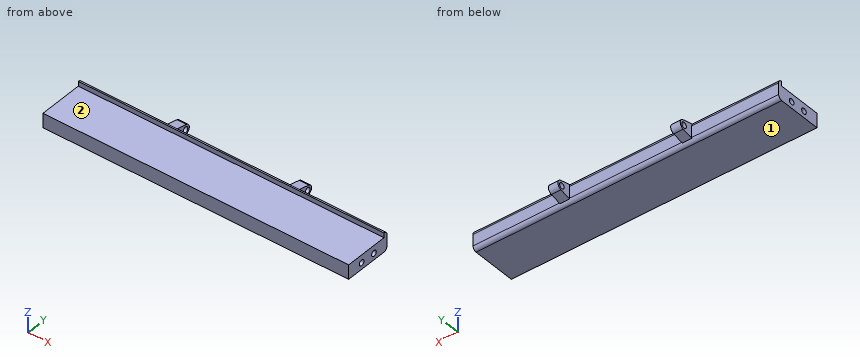
Autodesk Inventor part; units mm, degrees
ref_plane "Work Plane1" through (-8, -12.5, 0) normal (1, 0, 0) x (0, 0, -1)
ref_plane "Work Plane2" through (-40, -12.5, 0) normal (-1, 0, 0) x (0, 0, 1)
ref_plane "Work Plane3" through (20, 10.5, 6) normal (0, 0, -1) x (-1, 0, 0)
sketch "Sketch1" plane through (0, 0, 0) normal (0, 0, 1) x (1, 0, 0)
  line L0 (40, 12.5) -> (-40, 12.5)
  line L1 (-40, 12.5) -> (-40, -12.5)
  line L2 (-40, -12.5) -> (40, -12.5)
  line L3 (40, -12.5) -> (40, 12.5)
  line L4 (40, 12.5) -> (-40, -12.5) construction
  line L5 (-40, 12.5) -> (40, -12.5) construction
  point P0 (0, 0)
  dimension "d0" = 80
  dimension "d1" = 25
extrude "Extrusion1" add sketch "Sketch1" along normal blind 10
ref_plane "Work Plane1" through (-8, -12.5, 0) normal (1, 0, 0) x (0, 0, -1)
sketch "Sketch2" plane through (-8, -12.5, 0) normal (1, 0, 0) x (0, 0, -1)
  circle A0 centre (-5.3658, 30) radius 2.5
  line L0 (0, 25) -> (-10, 25)
  line L1 (-9.1092, 25) -> (-7.7995, 30.572)
  line L2 (-2.9321, 30.572) -> (-1.6224, 25)
  point P0 (0, 12.5)
  dimension "d5" = 5
  dimension "d11" = 5
extrude "Extrusion2" add sketch "Sketch2" along normal mid plane 5
sketch "Sketch3" plane through (-5.5, -12.5, 0) normal (1, 0, 0) x (0, 0, -1)
  arc A0 (-2.9321, 30.572) -> (-7.7995, 30.572) centre (-5.3658, 30) ccw
  circle A1 centre (-5.3658, 30) radius 1.5
  point P0 (0, 12.5)
  dimension "d8" = 3
extrude "Extrusion3" cut sketch "Sketch3" against normal blind 20
sketch "Sketch4" plane through (0, 0, 0) normal (0, 0, -1) x (-1, 0, 0)
  point P0 (0, 0)
sketch "Sketch5" plane through (-40, -12.5, 0) normal (-1, 0, 0) x (0, 0, 1)
  point P0 (0, 12.5)
ref_plane "Work Plane2" through (-40, -12.5, 0) normal (-1, 0, 0) x (0, 0, 1)
mirror "Mirror1" about plane through (-40, 12.5, 0) normal (-1, 0, 0) of "Extrusion2", "Extrusion1"
fillet "Fillet1" radius 2 2 edges at (-40, 12.5, 10) (-40, 12.5, 0)
sketch "Sketch6" plane through (-74.5, 17.5, 5.3658) normal (-1, 0, 0) x (0, 0, 1)
  circle A0 centre (0, 0) radius 1.5
  point P0 (-5.3658, -17.5)
extrude "Extrusion4" cut sketch "Sketch6" against normal blind 20
ref_plane "Work Plane3" through (20, 10.5, 6) normal (0, 0, -1) x (-1, 0, 0)
sketch "Sketch7" plane through (40, -12.5, 10) normal (1, 0, 0) x (0, 0, -1)
  circle A0 centre (6.606, 16.5) radius 1.5
  circle A1 centre (6.606, 8.5) radius 1.5
  line L0 (10, 0) -> (0, 0)
  line L1 (10, 0) -> (10, 23)
  point P0 (10, 12.5)
  point P1 (5, 0)
  dimension "d16" = 3
  dimension "d17" = 3
  dimension "d19" = 8.5
  dimension "d20" = 8
  dimension "d32" = 3.394
  dimension "d33" = 3.394
extrude "Extrusion5" cut sketch "Sketch7" against normal blind 8
ref_plane "Work Plane4" through (-120, -12.5, 0) normal (-1, 0, 0) x (0, 0, 1)
mirror "Mirror2" about plane through (-40, -12.5, 0) normal (-1, 0, 0) of "Extrusion5"
thread "Thread1"
thread "Thread2"
thread "Thread3"
thread "Thread4"
sketch "Sketch8" plane through (0, 0, 0) normal (0, 0, -1) x (-1, 0, 0)
  line L0 (-40, 10.5) -> (120, 10.5) construction
  line L1 (-40, -12.5) -> (-40, 10.5) construction
  line L2 (-40, -12.5) -> (120, -12.5) construction
  line L3 (120, -12.5) -> (120, 10.5)
  point P0 (0, 0)
sketch "Sketch9" plane through (0, 0, 10) normal (0, 0, 1) x (1, 0, 0)
  line L0 (-120, 10.5) -> (40, 10.5)
  line L1 (-120, -12.5) -> (-120, 10.5)
  line L2 (40, -12.5) -> (-120, -12.5)
  line L3 (40, -12.5) -> (40, 10.5)
  point P0 (0, 0)
extrude "Extrusion6" cut sketch "Sketch9" against normal blind 2.5
properties part number "plate"
Can you work these out from the model? Positions are in its coordinate system, mm. Face numbers are marked on the shaded views. A direction names the side the tool comes from. Coordinates: 2 decimals unless noted, no trailing zeros. Order: outer loops, then holes, each group sorted by start corner. A loop starts at its lowest first (then second) coordinate and runs counter-clockwise, first axis right, second up. Notation, with made-up numbers: (55.25, 84) - (103.25, 84) arc R20 ccw to (103.25, 94) - close; hole circle Ø10 at (-30.5, 49.25). An arc over 180 degrees is marked (long way). Answer as a JSON object with one key per item and string values. Group by question number.
Q1. Imagine slicing it at A-A (x = -30). Please give me the cut outline in (y, z).
Q2. Will these pins go through, and if not, where does the flat tip stop? P1, Ø6, axis at y = 16.5, z = 5, coming from the -X side; P2, Ø0.9, axis at y = -4, z = 3, coming from the -X side; P3, Ø1.8, axis at y = -4, z = 3.394, coming from the +X side.
Q3. On a 3-axis mill with a long thin cutter (end or side, diameter ignored), from which of +Z, -Z, +X, -X, +Y, -Y can I reach the whole of each face in a straight line? I mean the marked faces 1 and 2. Say none if no direction works.
Q4. I need wall thicknesses on line 1 (Z direction, x = -74.5, y = -9); line 2 (Z direction, x = -72, y = 17); line 3 (Y direction, x = -111, z = 6.5). Which ranges of each line are inside material? Lowest first, please. Write a range as from..to.
Q5. Imagine slicing it at B-B (y = -4). Please give me the cut outline in (x, z), and give its area (3 significant figures).
Q6. Imagine slicing it at C-C (x = -7). Please give me the cut outline in (y, z).
Determined:
{
 "1": {"outline": "(-12.5, 0) - (10.5, 0) arc R2 ccw to (12.5, 2) - (12.5, 8) arc R2 ccw to (10.5, 10) - (10.5, 7.5) - (-12.5, 7.5) - close"},
 "2": {"P1": "stops at x = -74.5", "P2": "stops at x = -112", "P3": "stops at x = 32"},
 "3": {"face 1": "-Z, +X, -X, +Y, -Y", "face 2": "+Z, +X, -X, -Y"},
 "4": {"line 1": "z = 0..7.5", "line 2": "z = 2.68..3.95, 6.78..8.05", "line 3": "y = -12.5..12.5"},
 "5": {"outline": "(-120, 0) - (40, 0) - (40, 1.89) - (32, 1.89) - (32, 4.89) - (40, 4.89) - (40, 7.5) - (-120, 7.5) - (-120, 4.89) - (-112, 4.89) - (-112, 1.89) - (-120, 1.89) - close", "area": "1,150 mm2"},
 "6": {"outline": "(-12.5, 0) - (10.5, 0) arc R2 ccw to (12.46, 1.61) - (18.07, 2.93) arc R2.5 ccw to (18.07, 7.8) - (12.1, 9.2) arc R2 ccw to (10.5, 10) - (10.5, 7.5) - (-12.5, 7.5) - close; hole circle Ø3 at (17.5, 5.37)"}
}
